from build123d import *

# Parameters (mm, degrees)
F0_R     = 1.5875
F1_DEPTH = 12.7
F2_SIZE  = 1.524
F3_R     = 2.38125
F4_DEPTH = 2.38125
F5_W     = 1.5875
F5_H     = 0.79375
F5_W_2   = 0.79375
F5_H_2   = 1.5875
F6_DEPTH = 1.5875


# Not quite as in the source:
# - a fillet or chamfer that OpenCascade refuses, or shapes differently, is made with other operations: its cross-section is extruded or revolved along the edge and cut away or added


with BuildPart() as f1:
    # F0 (on Top) → F1 (new body)
    with BuildSketch(Plane.XY):
        Circle(F0_R)
    extrude(amount=F1_DEPTH)

    # F2
    f2_edges = [f1.edges().sort_by_distance(p)[0] for p in [
        (-1.5875, 0, 0),
    ]]
    chamfer(f2_edges, length=F2_SIZE)

    # F3 (on face) → F4 (join)
    with BuildSketch(Plane.XY.offset(12.7)):
        Circle(F3_R)
    extrude(amount=F4_DEPTH)

    # F5 (on face) → F6 (cut)
    with BuildSketch(Plane.XY.offset(15.08125)):
        with Locations((0, 1.190625)):
            Rectangle(F5_W, F5_H)
        with Locations((1.190625, 0)):
            Rectangle(F5_W_2, F5_H_2)
        Rectangle(F5_W, F5_H_2)
        with Locations((-1.190625, 0)):
            Rectangle(F5_W_2, F5_H_2)
        with Locations((0, -1.190625)):
            Rectangle(F5_W, F5_H)
    extrude(amount=-F6_DEPTH, mode=Mode.SUBTRACT)

    # F7: fillet of radius 1.27 on 1 edges, made by hand

    # F7_s1 → F7_t2 (revolve, cut)
    with BuildSketch(Plane.XZ):
        with BuildLine():
            ThreePointArc((2.38125, 13.81125), (2.0092756121, 14.7092756121), (1.11125, 15.08125))
            Line((1.11125, 15.08125), (2.38125, 15.08125))
            Line((2.38125, 15.08125), (2.38125, 13.81125))
        make_face()
    revolve(axis=Axis((0, 0, 15.08125), (0, 0, 1)), mode=Mode.SUBTRACT)


solid = f1.part
Build history of the part. All positions in model axes, mm. A direction names the side the tool comes from. Coordinates: 2 decimals unless noted, no trailing zeros. Write each loop counter-clockwise with the first axis right and the second up, starting at its lowest first coordinate (ties: lowest second). Pieces come first, ordered by that corner, then holes. Notation, with made-up numbers: (-10.5, 58) -> (31.5, 58) arc R22 ccw to (31.5, 95) -> close; hole circle Ø8 at (71, -27). An arc over 180 degrees is marked (long way). Use CSV: the item, a comma, the result in double quotes. Start each with the question number.
Q1. Pull direction Y, two halves, no side cores. Call faces 3 (the flat face through (0, 0, 13.494)), 4 (the flat face through (0, -2, 12.7)), 5 (the cylindrical face through (-0.34, -1.55, 7.03)): released by +Y, released by -Y, zero draft, split by the parting line, or undercut.
Q2. Cut at B-B, the plane z = 13. List the corners of the cut face in (x, y), then the cut area to 3 significant figures.
Q3. Drill centre lines: probe 1 along X at (y, z) = (0.1, 2.25); probe 2 along X at (y, z) = (-0.4, 14); probe 3 along X at (y, z) = (0.5, 1). Where is each one in solid material? Low to high.
Q4. Cut at A-A, the plane z = 9. List the corners of the cut face in (x, y) (1 decimal).
Q5. Flat gauge pins, fed straight in: pin 1 Ø0.6 at (x, z) = (-1, 14.5) entering from +Y; pin 2 Ø0.9 at (x, z) = (1, 14.5) entering from +Y; pin 3 Ø0.7 at (y, z) = (0.5, 14.5) entering from -X. Where does each tip first touch, or does it go through?
Q6. 3-axis set-ups, long thin cutter, end or side, ignore diameter. For faces 1 (the cylindrical face through (-1.89, -1.45, 13.25)), 2 (the flat face through (0, -1.588, 14)): which of +Z, -Z, +X, -X, +Y, -Y reach the whole face in a straight line?
Checked values:
1,face 3,"undercut"
1,face 4,"zero draft"
1,face 5,"split by the parting line"
2,outline,"circle Ø4.76 at (0, 0)"
2,area,"17.8 mm²"
3,probe 1,"x = -1.58 to 1.58"
3,probe 2,"x = -2.33 to -1.59, 1.59 to 2.33"
3,probe 3,"x = -0.94 to 0.94"
4,outline,"circle Ø3.2 at (0, 0)"
5,pin 1,"stops at y = 2.15"
5,pin 2,"stops at y = 2.22"
5,pin 3,"stops at x = -2.3"
6,face 1,"+Z, -Z"
6,face 2,"+Z"
